Here's how the part is built. I have some questions about the finished solid (model axes, mm). A direction names the side the tool comes from. Give positions to 0.01 mm unless a question says otherwise; leave off trailing zeros. Loops run counter-clockwise (first coordinate to the right, second up) from the corner with the lowest first, then second, coordinate; pieces in that order, holes last. Notation, with made-up numbers: (44.5, 6) - (69.5, 6) arc R19 ccw to (69.5, 43) - close; hole circle Ø1 at (31.25, 11.25). An arc over 180 degrees is marked (long way). Use a Markdown table: item, result.
from build123d import *

# Parameters (mm, degrees)
SKETCH2_R                = 20.5
SKETCH2_R_2              = 17.5
BOSS_EXTRUDE1_DEPTH      = 35
SKETCH3_OUTSIDE_W        = 56.546
SKETCH3_OUTSIDE_H        = 56.546
CUT_EXTRUDE1_DEPTH       = 36
SKETCH5_R                = 2
CUT_EXTRUDE2_DEPTH       = 21.5
BOSS_EXTRUDE2_DEPTH      = 2.5
BOSS_EXTRUDE2_DEPTH_BACK = 2.5
SKETCH10_R               = 2.5
CUT_EXTRUDE3_DEPTH       = 16.0000001
FILLET2_R                = 2


with BuildPart() as part:
    # Sketch2 → Boss-Extrude1 (new body)
    with BuildSketch(Plane(origin=(0, 0, 0), x_dir=(1, 0, 0), z_dir=(0, 1, 0))):
        Circle(SKETCH2_R)
        Circle(SKETCH2_R_2, mode=Mode.SUBTRACT)
    extrude(amount=BOSS_EXTRUDE1_DEPTH)

    # Sketch3 outside → Cut-Extrude1 (cut, through all)
    with BuildSketch(Plane(origin=(0, 35, 0), x_dir=(1, 0, 0), z_dir=(0, 1, 0))):
        Rectangle(SKETCH3_OUTSIDE_W, SKETCH3_OUTSIDE_H)
        with BuildLine():
            Line((0, 0), (12.5, 16.248076809))
            ThreePointArc((12.5, 16.248076809), (0, 20.5), (-12.5, 16.248076809))
            Line((-12.5, 16.248076809), (0, 0))
        make_face(mode=Mode.SUBTRACT)
    extrude(amount=-CUT_EXTRUDE1_DEPTH, mode=Mode.SUBTRACT)

    # Sketch5 → Cut-Extrude2 (cut, through all)
    with BuildSketch(Plane.XY):
        with Locations((0, 30)):
            Circle(SKETCH5_R)
        with Locations((0, 5)):
            Circle(SKETCH5_R)
    extrude(amount=-CUT_EXTRUDE2_DEPTH, mode=Mode.SUBTRACT)

    # Sketch7 → Boss-Extrude2 (add, two sides)
    with BuildSketch(Plane(origin=(0, 15, 0), x_dir=(0, 1, 0), z_dir=(-1, 0, 0))) as boss_extrude2_sk:
        with BuildLine():
            Line((-2.5, 34.5), (-2.5, 18.5))
            Line((-2.5, 18.5), (7.5, 18.5))
            Line((7.5, 18.5), (7.5, 34.5))
            ThreePointArc((7.5, 34.5), (2.5, 39.5), (-2.5, 34.5))
        make_face()
    extrude(amount=BOSS_EXTRUDE2_DEPTH)
    extrude(boss_extrude2_sk.sketch, amount=-BOSS_EXTRUDE2_DEPTH_BACK)

    # Sketch10 → Cut-Extrude3 (cut, through all)
    with BuildSketch(Plane(origin=(-2.5, 0, 0), x_dir=(0, 1, 0), z_dir=(-1, 0, 0))):
        with Locations((17.5, 34.5)):
            Circle(SKETCH10_R)
    extrude(amount=-CUT_EXTRUDE3_DEPTH, mode=Mode.SUBTRACT)

    # Fillet2
    fillet2_edges = [part.edges().sort_by_distance(p)[0] for p in [
        (-2.5, 17.5, -20.346989949),
        (0, 12.5, -20.5),
        (0, 22.5, -20.5),
        (2.5, 17.5, -20.346989949),
    ]]
    fillet(fillet2_edges, radius=FILLET2_R)


solid = part.part
(1) Suppose I cut it at D-D on y = 13. Write out the boundary of the cut face in (x, z).
A:
| item | result |
|---|---|
| outline | (-12.5, -16.25) arc R20.5 ccw to (-4.1, -20.09) arc R2 cw to (-2.5, -22.05) - (-2.5, -36.68) - (2.5, -36.68) - (2.5, -22.05) arc R2 cw to (4.1, -20.09) arc R20.5 ccw to (12.5, -16.25) - (10.67, -13.87) arc R17.5 cw to (-10.67, -13.87) - close |
(2) We'd pull the mould along Z, two halves only. Please class faces 4 (the face through (-2.96, 17.4, -20.77)), 5 (the face through (0.2, 17.3, -17.5)), 6 (the face through (0, 28, -19)), 7 (the face through (-0.04, 15.66, -36.19)): pulls with the +Z half, pulls with the -Z half, needs draft (parallel to the pull), parting line crosses it, or undercut.
A:
| item | result |
|---|---|
| face 4 | pulls with the -Z half |
| face 5 | pulls with the +Z half |
| face 6 | needs draft |
| face 7 | undercut |
(3) Will these pins go through, and if not, where does the flat tip stop? pin 1 (5 mm diameter, centred on y = 11, z = -35, fed in from -X); pin 2 (2.5 mm diameter, centred on x = 0, z = -30.5, fed in from -Y); pin 3 (10 mm diameter, centred on x = 1, y = 7, fed in from -Z); pin 4 (3 mm diameter, centred on x = 0, y = 5, fed in from -Z).
A:
| item | result |
|---|---|
| pin 1 | x = -2.5 |
| pin 2 | y = 12.5 |
| pin 3 | z = -21.16 |
| pin 4 | through |
(4) On a 3-axis mill with a long thin cutter (end or side, diameter ignored), from which of +Z, -Z, +X, -X, +Y, -Y can I reach the whole of each face in a straight line? I mean faces 1 (the face through (-2.5, 17, -29)), 2 (the face through (2.5, 17, -29)), 3 (the face through (0, 12.5, -29)). Say none if no direction works.
A:
| item | result |
|---|---|
| face 1 | -Z, -X, +Y, -Y |
| face 2 | -Z, +X, +Y, -Y |
| face 3 | -Z, +X, -X, -Y |
(5) Suppose I cut it at C-C on z = -26.5. Write out the boundary of the cut face in (x, y), plus the area to 3 significant figures.
A:
| item | result |
|---|---|
| outline | (-2.5, 12.5) - (2.5, 12.5) - (2.5, 22.5) - (-2.5, 22.5) - close |
| area | 50.0 mm2 |
(6) Suppose I cut it at A-A on x = 0. Write out the boundary of the cut face in (y, z), plus the area to 3 significant figures.
A:
| item | result |
|---|---|
| outline | (0, -20.5) - (3, -20.5) - (3, -17.5) - (0, -17.5) - close; (7, -20.5) - (10.5, -20.5) arc R2 cw to (12.5, -22.5) - (12.5, -34.5) arc R5 ccw to (22.5, -34.5) - (22.5, -22.5) arc R2 cw to (24.5, -20.5) - (28, -20.5) - (28, -17.5) - (7, -17.5) - close; (32, -20.5) - (35, -20.5) - (35, -17.5) - (32, -17.5) - close; hole circle Ø5 at (17.5, -34.5) |
| area | 242 mm2 |
(7) If I drill on line 1 (Y direction, x = 0, z = -18.5); line 2 (Z direction, x = 0.5, y = 17.5); line 3 (X direction, y = 30, z = -18.05), over which ranges is the centre line in solid material (lowest first)?
A:
| item | result |
|---|---|
| line 1 | 0 to 3, 7 to 28, 32 to 35 |
| line 2 | -39.5 to -37, -32 to -17.49 |
| line 3 | -9.72 to -2, 2 to 9.72 |
(8) Suppose I cut it at B-B on y = 17.5. Write out the boundary of the cut face in (x, z).
A:
| item | result |
|---|---|
| outline | (-12.5, -16.25) arc R20.5 ccw to (-4.1, -20.09) arc R2 cw to (-2.5, -22.05) - (-2.5, -32) - (2.5, -32) - (2.5, -22.05) arc R2 cw to (4.1, -20.09) arc R20.5 ccw to (12.5, -16.25) - (10.67, -13.87) arc R17.5 cw to (-10.67, -13.87) - close; (-2.5, -39.5) - (2.5, -39.5) - (2.5, -37) - (-2.5, -37) - close |
